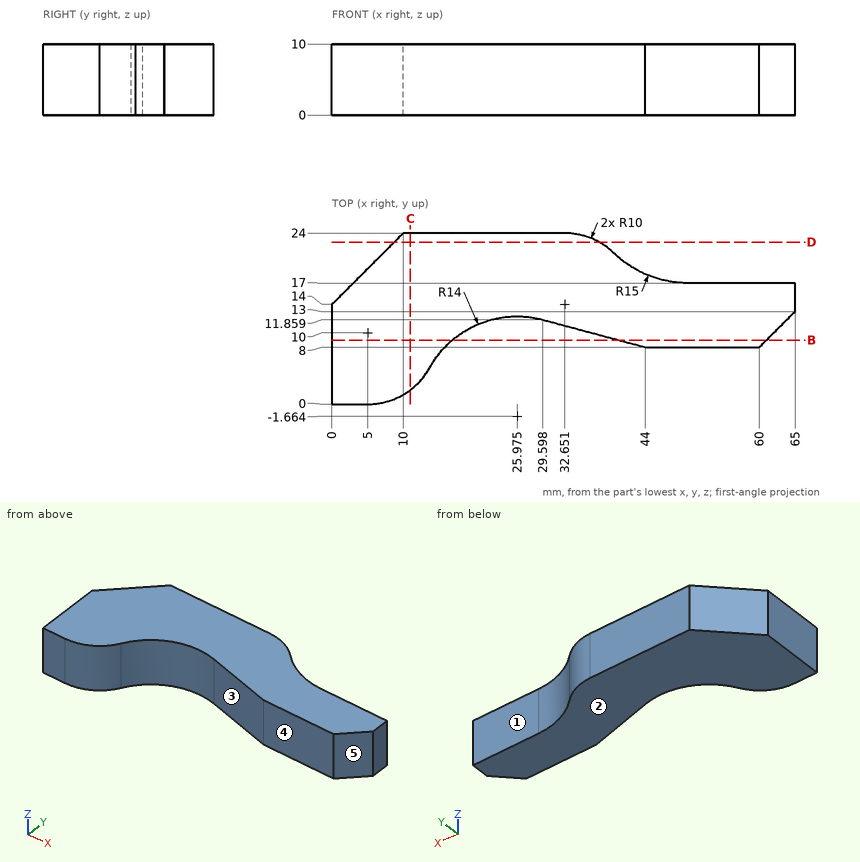
Input: dimensioned drawing with shaded views. Units: mm. Origin: part minimum x, y, z. A direction names the side the tool comes from. Give positions to 0.01 mm unless a question says otherwise; leave off trailing zeros. Loops run counter-clockwise (first coordinate to the right, second up) from the corner with the lowest first, then second, coordinate; pieces in that order, holes last. Notation, with made-up numbers: (25.25, 84.5) -> (76.25, 84.5) arc R23 cw to (76.25, 98.5) -> close; hole circle Ø6 at (37, -34.75). An arc over 180 degrees is marked (long way). Use a Markdown table: item, result. Add a question column.
1) Section query B-B, the plane y = 9. Return the cut outline in (x, z) (1 decimal).
2) Reachability of the marked faces 1 and 2 from +Z, -Z, +X, -X, +Y, -Y: full face, straight path, thin tool, end or side. Return the list, or none.
3) First-contact query: pin 1 (3 mm diameter, centred on x = 61, z = 4.5, fed in from +Y); pin 2 (1 mm diameter, centred on x = 33.5, z = 7.5, fed in from +Y); pin 3 (4 mm diameter, centred on x = 36.5, z = 6, fed in from -Y); pin 4 (3 mm diameter, centred on x = 24, y = 11.5, fed in from -Z). Flat tips, straight axial feed; report the tip coordinate or a pass-through.
4) Section query D-D, the plane y = 22.75. Return the cut outline in (x, z), then the cut area to 3 significant figures.
5) Line query: line 1 along Y through (x, z) = (62, 3.75); line 2 along Y through (x, z) = (51, 1.25); line 3 along X through (y, z) = (4.25, 8). Output: solid intervals per line, ascending. Write a range as [from, to].
6) Pull-direction query (X, two-part tool) for the marked faces 3, 4 and 5; classes: +X half, -X half, draft (parallel to the pull), parting line (faces both ways), or undercut.
7) Section query C-C, the plane x = 11. Return the cut outline in (y, z).
Numbers:
| question | item | result |
|---|---|---|
| 1 | outline | (0, 0) -> (16.9, 0) -> (16.9, 10) -> (0, 10) -> close; (40.3, 0) -> (61, 0) -> (61, 10) -> (40.3, 10) -> close |
| 2 | face 1 | +Z, -Z, +X, +Y |
| 2 | face 2 | -Z, +X, -X, +Y, -Y |
| 3 | pin 1 | stops at y = 17 |
| 3 | pin 2 | stops at y = 23.99 |
| 3 | pin 3 | stops at y = 9.47 |
| 3 | pin 4 | stops at z = 0 |
| 4 | outline | (8.75, 0) -> (37.49, 0) -> (37.49, 10) -> (8.75, 10) -> close |
| 4 | area | 287 mm2 |
| 5 | line 1 | y = [10, 17] |
| 5 | line 2 | y = [8, 17] |
| 5 | line 3 | x = [0, 13.18] |
| 6 | face 3 | undercut |
| 6 | face 4 | draft |
| 6 | face 5 | +X half |
| 7 | outline | (2, 0) -> (24, 0) -> (24, 10) -> (2, 10) -> close |
